Here's how the part is built. I have some questions about the finished solid (model axes, mm). A direction names the side the tool comes from. Round coordinates to 2 decimals unless told otherwise and drop trailing zeros. Order: outer loops, then holes, each group sorted by start corner. A loop starts at its lowest first (then second) coordinate and runs counter-clockwise, first axis right, second up. Notation, with made-up numbers: (3, 23.25) -> (57, 23.25) arc R11 cw to (57, 27.25) -> close; hole circle Ø8 at (51.5, -6.75). An arc over 180 degrees is marked (long way). Use a Markdown table: item, result. Add a question column.
from build123d import *

# Parameters (mm, degrees)
F1_R     = 2.85
F1_R_2   = 1.1
F2_DEPTH = 1.2
F3_R     = 4
F4_SIZE  = 0.9


with BuildPart() as f2:
    # F1 (on Top) → F2 (new body)
    with BuildSketch(Plane.XY):
        with BuildLine():
            Line((-8.5, -7.988706), (-19.519778, -19.779415))
            ThreePointArc((-19.519778, -19.779415), (-24.064093, -28.302939), (-15.866839, -23.193508))
            Line((-15.866839, -23.193508), (-5.078098, -11.65))
            Line((-5.078098, -11.65), (5.078098, -11.65))
            Line((5.078098, -11.65), (15.866839, -23.193508))
            ThreePointArc((15.866839, -23.193508), (24.064093, -28.302939), (19.519778, -19.779415))
            Line((19.519778, -19.779415), (8.5, -7.988706))
            Line((8.5, -7.988706), (8.5, 0.657413))
            Line((8.5, 0.657413), (20.458776, 19.653658))
            ThreePointArc((20.458776, 19.653658), (23.313776, 28.881347), (16.227429, 22.317434))
            Line((16.227429, 22.317434), (5.545858, 5.35))
            Line((5.545858, 5.35), (-5.545858, 5.35))
            Line((-5.545858, 5.35), (-16.227429, 22.317434))
            ThreePointArc((-16.227429, 22.317434), (-23.313776, 28.881347), (-20.458776, 19.653658))
            Line((-20.458776, 19.653658), (-8.5, 0.657413))
            Line((-8.5, 0.657413), (-8.5, -7.988706))
        make_face()
        with Locations((-20.65, -24.65)):
            Circle(F1_R, mode=Mode.SUBTRACT)
        with Locations((-4.5, -7.65)):
            Circle(F1_R_2, mode=Mode.SUBTRACT)
        with Locations((20.65, -24.65)):
            Circle(F1_R, mode=Mode.SUBTRACT)
        with Locations((4.5, -7.65)):
            Circle(F1_R_2, mode=Mode.SUBTRACT)
        with Locations((-4.5, 1.35)):
            Circle(F1_R_2, mode=Mode.SUBTRACT)
        with Locations((-20.65, 24.65)):
            Circle(F1_R, mode=Mode.SUBTRACT)
        with Locations((4.5, 1.35)):
            Circle(F1_R_2, mode=Mode.SUBTRACT)
        with Locations((20.65, 24.65)):
            Circle(F1_R, mode=Mode.SUBTRACT)
    extrude(amount=F2_DEPTH)

    # F3
    f3_edges = [f2.edges().sort_by_distance(p)[0] for p in [
        (-5.545858, 5.35, 0.6),
        (5.545858, 5.35, 0.6),
        (-16.227429, 22.317434, 0.6),
        (-20.458776, 19.653658, 0.6),
        (16.227429, 22.317434, 0.6),
        (20.458776, 19.653658, 0.6),
        (8.5, 0.657413, 0.6),
        (8.5, -7.988706, 0.6),
        (19.519778, -19.779415, 0.6),
        (15.866839, -23.193508, 0.6),
        (5.078098, -11.65, 0.6),
        (-5.078098, -11.65, 0.6),
        (-15.866839, -23.193508, 0.6),
        (-8.5, 0.657413, 0.6),
        (-8.5, -7.988706, 0.6),
        (-19.519778, -19.779415, 0.6),
    ]]
    fillet(f3_edges, radius=F3_R)

    # F4
    f4_edges = [f2.edges().sort_by_distance(p)[0] for p in [
        (-5.6, 1.35, 1.2),
        (3.4, 1.35, 1.2),
        (3.4, -7.65, 1.2),
        (-5.6, -7.65, 1.2),
    ]]
    chamfer(f4_edges, length=F4_SIZE)


solid = f2.part
(1) If we mould it in two halves opening along X, with no side actions, what happens to faces 5 (the cylindrical face through (21.965, -27.178, 0.592)), 6 (the cylindrical face through (-19.44, -19.28, 0.61)), 7 (the flat face through (2, -2, 0))? For each: pulls with the +X half, pulls with the -X half, needs draft (parallel to the pull), parting line crosses it, or undercut.
(2) I want a section at B-B on y = 9. List the corners of the cut face in (x, z) for me.
(3) Please list where these lines run through material, in increasing order: probe 1 along Y at (x, z) = (-21, 0.8); probe 2 along Y at (x, z) = (4.5, 0.25); probe 3 along X at (y, z) = (25, 0.8). Write a range as from..to.
(4) I want a section at A-A on x = -11.5. List the corners of the cut face in (y, z) for me.
(5) I want a section at D-D on z = 0.65. State how many separate pieces and enclosed holes the cut face has, and give its area (3 significant figures).
(6) I want a section at C-C on y = -7.65. List the corners of the cut face in (x, z) for me.
(7) I'm going to push flat-ended pins straight in: P1, Ø5, axis at x = -20.65, y = -24.65, coming from the -Z side; P2, Ø0.6, axis at x = -0.5, z = 0.5, coming from the +Y side. Where does each tip first touch, or does it pass through?
(8) On a 3-axis mill with a long thin cutter (end or side, diameter ignored), from which of +Z, -Z, +X, -X, +Y, -Y can I reach the whole of each face in a straight line? I mean faces 1 (the cylindrical face through (8.652, 0.597, 0.608)), 2 (the cylindrical face through (-15.772, 22.15, 0.608)), 3 (the cylindrical face through (5.246, 5.835, 0.608)), 4 (the flat face through (-10.48, -17.43, 0.59)). Say none if no direction works.
Output:
| question | item | result |
|---|---|---|
| 1 | face 5 | undercut |
| 1 | face 6 | pulls with the -X half |
| 1 | face 7 | needs draft |
| 2 | outline | (-13.75, 0) -> (-7.84, 0) -> (-7.84, 1.2) -> (-13.75, 1.2) -> close; (7.84, 0) -> (13.75, 0) -> (13.75, 1.2) -> (7.84, 1.2) -> close |
| 3 | probe 1 | -29.64..-27.48, -21.82..-19.66, 19.47..21.82, 27.48..29.64 |
| 3 | probe 2 | -11.82..-8.75, -6.55..0.25, 2.45..5.52 |
| 3 | probe 3 | -25.64..-23.48, -17.82..-15.66, 15.66..17.82, 23.48..25.64 |
| 4 | outline | (-18.52, 0) -> (-11.2, 0) -> (-11.2, 1.2) -> (-18.52, 1.2) -> close; (5.42, 0) -> (14.81, 0) -> (14.81, 1.2) -> (5.42, 1.2) -> close |
| 5 | separate pieces | 1 |
| 5 | enclosed holes | 8 |
| 5 | area | 818 mm² |
| 6 | outline | (-8.7, 0) -> (-5.6, 0) -> (-5.6, 0.3) -> (-6.5, 1.2) -> (-8.7, 1.2) -> close; (-3.4, 0) -> (3.4, 0) -> (3.4, 0.3) -> (2.5, 1.2) -> (-2.5, 1.2) -> (-3.4, 0.3) -> close; (5.6, 0) -> (8.7, 0) -> (8.7, 1.2) -> (6.5, 1.2) -> (5.6, 0.3) -> close |
| 7 | P1 | through |
| 7 | P2 | y = 5.35 |
| 8 | face 1 | +Z, -Z, +X |
| 8 | face 2 | +Z, -Z |
| 8 | face 3 | +Z, -Z, +Y |
| 8 | face 4 | +Z, -Z, -Y |
